The figure shows three views and two pictorial views of one solid part (mm, origin at its lowest corner). Answer the questions. Round coordinates to 2 decimals unless told otherwise and drop trailing zeros. Write each loop counter-clockwise with the first axis right and the second up, starting at its lowest first coordinate (ties: lowest second). Pieces come first, ordered by that corner, then holes.
Item 1: Find section C-C on y = 2.35. Give the vertices of the cut face in (x, z), then the cut area to 3 significant figures.
Item 2: Find section A-A on z = 48.3. Give the vertices of the cut face in (x, y), then the cut area to 3 significant figures.
Item 3: Find the intervals of material crossed by probe 1 along Z at (x, y) = (20.8, 0.6); probe 2 along X at (y, z) = (0.9, 20.8), in increasing order.
Item 4: Each of these flat-tipped pins is pushed along its axis until it touches: pin 1 (0.9 mm diameter, centred on x = 51, y = 2, fed in from -Z); pin 2 (6 mm diameter, centred on x = 51.5, z = 58, fed in from +Y); pin 3 (0.9 mm diameter, centred on x = 46, y = 1.5, fed in from +Z); pin 4 (1.7 mm diameter, centred on x = 20.8, z = 20.8, fed in from -Y). Where does it stop, or does it pass through?
Item 5: Find section D-D on x = 75.8. Give the vertices of the cut face in (y, z).
Item 6: Find section B-B on x = 48.3. Give the vertices of the cut face in (y, z), then the cut area to 3 significant figures.
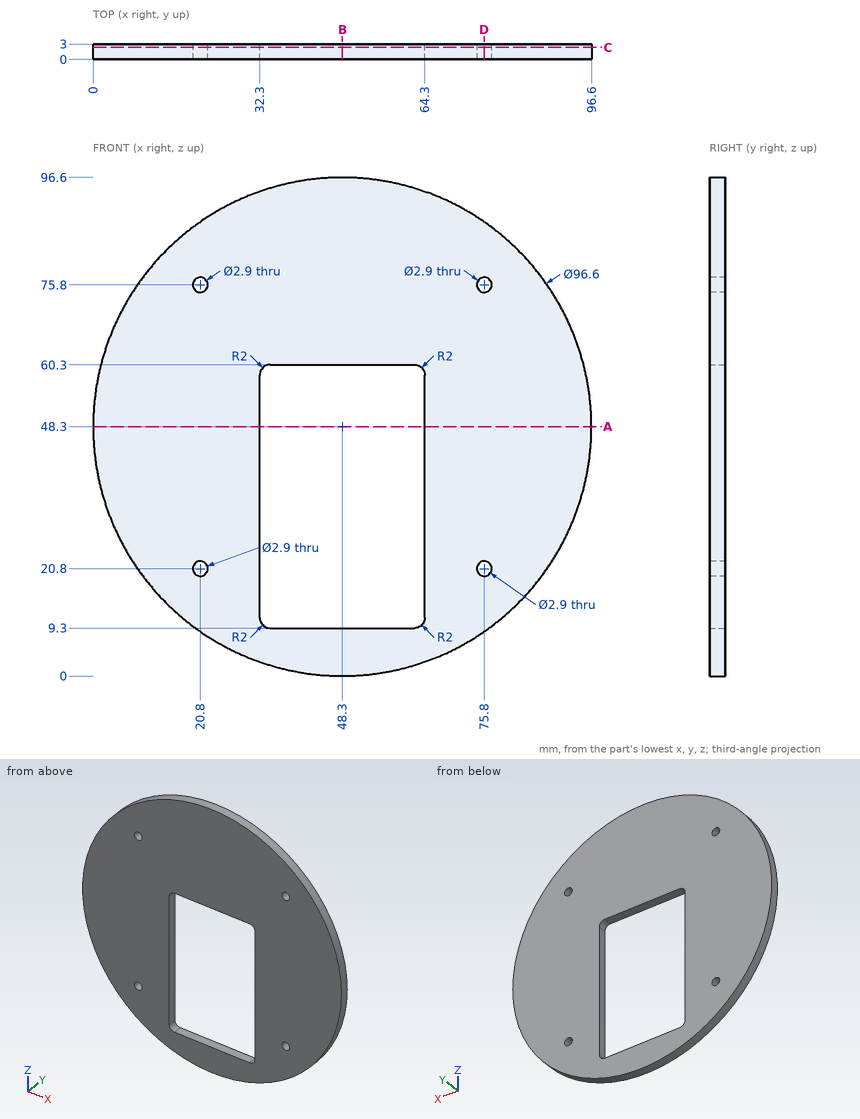
Check values:
1. outline: circle Ø96.6 at (48.3, 48.3); hole circle Ø2.9 at (20.8, 20.8); hole circle Ø2.9 at (20.8, 75.8); hole (32.3, 11.3) arc R2 ccw to (34.3, 9.3) - (62.3, 9.3) arc R2 ccw to (64.3, 11.3) - (64.3, 58.3) arc R2 ccw to (62.3, 60.3) - (34.3, 60.3) arc R2 ccw to (32.3, 58.3) - close; hole circle Ø2.9 at (75.8, 20.8); hole circle Ø2.9 at (75.8, 75.8)
1. area: 5,670 mm2
2. outline: (0, 0) - (32.3, 0) - (32.3, 3) - (0, 3) - close; (64.3, 0) - (96.6, 0) - (96.6, 3) - (64.3, 3) - close
2. area: 194 mm2
3. probe 1: z = 8.59 to 19.35, 22.25 to 74.35, 77.25 to 88.01
3. probe 2: x = 8.59 to 19.35, 22.25 to 32.3, 64.3 to 74.35, 77.25 to 88.01
4. pin 1: stops at z = 0.05
4. pin 2: stops at y = 3
4. pin 3: stops at z = 96.56
4. pin 4: passes through
5. outline: (0, 8.59) - (3, 8.59) - (3, 19.35) - (0, 19.35) - close; (0, 22.25) - (3, 22.25) - (3, 74.35) - (0, 74.35) - close; (0, 77.25) - (3, 77.25) - (3, 88.01) - (0, 88.01) - close
6. outline: (0, 0) - (3, 0) - (3, 9.3) - (0, 9.3) - close; (0, 60.3) - (3, 60.3) - (3, 96.6) - (0, 96.6) - close
6. area: 137 mm2
